from build123d import *

# Parameters (mm, degrees)
SKETCH1_W           = 40.9
SKETCH1_H           = 26.8
BOSS_EXTRUDE1_DEPTH = 10
SKETCH2_W           = 54
SKETCH2_H           = 20
BOSS_EXTRUDE2_DEPTH = 3
SKETCH3_R           = 1.5
CUT_EXTRUDE1_DEPTH  = 3
SKETCH4_W           = 40.9
SKETCH4_H           = 20
BOSS_EXTRUDE3_DEPTH = 3
BOSS_EXTRUDE4_DEPTH = 4.2
SKETCH6_R           = 2.5
BOSS_EXTRUDE5_DEPTH = 5


with BuildPart() as part:
    # Sketch1 → Boss-Extrude1 (new, symmetric)
    with BuildSketch(Plane.XY):
        Rectangle(SKETCH1_W, SKETCH1_H)
    extrude(amount=BOSS_EXTRUDE1_DEPTH, both=True)

    # Sketch2 → Boss-Extrude2 (add)
    with BuildSketch(Plane(origin=(0, 13.4, 0), x_dir=(1, 0, 0), z_dir=(0, 1, 0))):
        Rectangle(SKETCH2_W, SKETCH2_H)
    extrude(amount=BOSS_EXTRUDE2_DEPTH)

    # Sketch3 → Cut-Extrude1 (cut)
    with BuildSketch(Plane(origin=(0, 16.4, 0), x_dir=(1, 0, 0), z_dir=(0, 1, 0))):
        with Locations(Location((-24, 0, 0), (0, 0, 180))):
            Circle(SKETCH3_R)
        with Locations(Location((24, 0, 0), (0, 0, 180))):
            Circle(SKETCH3_R)
    extrude(amount=-CUT_EXTRUDE1_DEPTH, mode=Mode.SUBTRACT)

    # Sketch4 → Boss-Extrude3 (add)
    with BuildSketch(Plane(origin=(0, 16.4, 0), x_dir=(1, 0, 0), z_dir=(0, 1, 0))):
        Rectangle(SKETCH4_W, SKETCH4_H)
    extrude(amount=BOSS_EXTRUDE3_DEPTH)

    # Sketch5 → Boss-Extrude4 (add)
    with BuildSketch(Plane(origin=(0, 19.4, 0), x_dir=(1, 0, 0), z_dir=(0, 1, 0))):
        with BuildLine():
            ThreePointArc((0.870933014, -2.870797047), (20.45, 0), (0.870933014, 2.870797047))
            ThreePointArc((0.870933014, 2.870797047), (-3, 0), (0.870933014, -2.870797047))
        make_face()
    extrude(amount=BOSS_EXTRUDE4_DEPTH)

    # Sketch6 → Boss-Extrude5 (add)
    with BuildSketch(Plane(origin=(0, 23.6, 0), x_dir=(1, 0, 0), z_dir=(0, 1, 0))):
        with Locations(Location((10.45, 0, 0), (0, 0, 270))):
            Circle(SKETCH6_R)
    extrude(amount=BOSS_EXTRUDE5_DEPTH)


solid = part.part
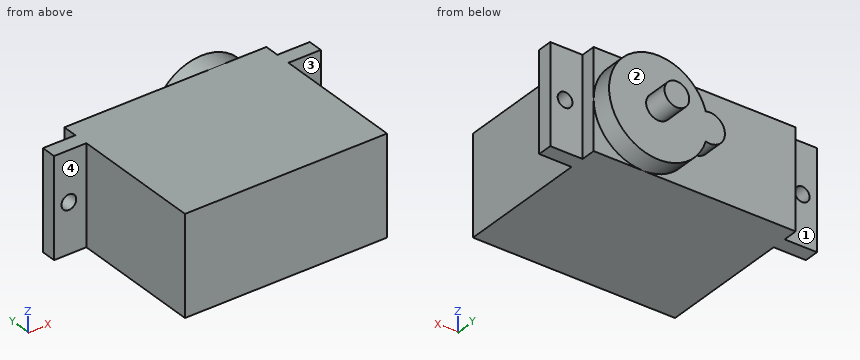
Can you work these out from the model? Positions are in its coordinate system, mm. Face numbers are marked on the shaded views. A direction names the side the tool comes from. Round coordinates to 2 decimals unless told otherwise and drop trailing zeros. Write each loop counter-clockwise with the first axis right and the second up, starting at its lowest first coordinate (ties: lowest second). Pieces come first, ordered by that corner, then holes. Notation, with made-up numbers: (-34, 84.5) -> (14, 84.5) arc R26 cw to (14, 99.5) -> close; hole circle Ø5 at (-23.75, -39.5). An arc over 180 degrees is marked (long way). One line per question, with ' | ' between items. Start each with the question number.
1) Suppose I cut it at D-D on y = 7. Write out the boundary of the cut face in (x, z), then the cut area to 3 significant figures.
2) I need wall thicknesses on line 1 (Z direction, x = 24, y = 14.95); line 2 (Y direction, x = 12, z = 4); line 3 (Y direction, x = 20, z = 9). Which ranges of each line are inside material? Lowest first, please. Write a range as [from, to].
3) I'm going to push flat-ended pins straight in: P1, Ø10, axis at y = 21, z = -1.5, coming from the +X side; P2, Ø7, axis at x = -25, z = -3.5, coming from the -Y side; P3, Ø5, axis at x = -22.5, z = 0, coming from the +Y side; P4, Ø0.9, axis at y = 17.5, z = 4.5, coming from the +X side. Where does each tip first touch, or does it pass through?
4) Suppose I cut it at A-A on x = 24. Write out the boundary of the cut face in (y, z), then the cut area to 3 significant figures.
5) Suppose I cut it at B-B on z = 4.75. Write out the boundary of the cut face in (x, y).
6) On a 3-axis mill with a long thin cutter (end or side, diameter ignored), from which of +Z, -Z, +X, -X, +Y, -Y can I reach the whole of each face in a straight line? I mean the marked faces 1, 2, 3 and 4. Say none if no direction works.
7) Suppose I cut it at C-C on x = 0. Write out the boundary of the cut face in (y, z), then the cut area to 3 significant figures.
Return value:
1) outline: (-20.45, -10) -> (20.45, -10) -> (20.45, 10) -> (-20.45, 10) -> close | area: 818 mm2
2) line 1: z = [-10, -1.5], [1.5, 10] | line 2: y = [-13.4, 23.6] | line 3: y = [-13.4, 19.4]
3) P1: stops at x = 27 | P2: stops at y = 13.4 | P3: stops at y = 19.4 | P4: stops at x = 20.45
4) outline: (13.4, -10) -> (16.4, -10) -> (16.4, -1.5) -> (13.4, -1.5) -> close; (13.4, 1.5) -> (16.4, 1.5) -> (16.4, 10) -> (13.4, 10) -> close | area: 51.0 mm2
5) outline: (-27, 13.4) -> (-20.45, 13.4) -> (-20.45, -13.4) -> (20.45, -13.4) -> (20.45, 13.4) -> (27, 13.4) -> (27, 16.4) -> (20.45, 16.4) -> (20.45, 19.4) -> (19.25, 19.4) -> (19.25, 23.6) -> (1.65, 23.6) -> (1.65, 19.4) -> (-20.45, 19.4) -> (-20.45, 16.4) -> (-27, 16.4) -> close
6) face 1: +Z, -Z, -X, +Y | face 2: +Y | face 3: +Z, -Z, +X, -Y | face 4: +Z, -Z, -X, -Y
7) outline: (-13.4, -10) -> (19.4, -10) -> (19.4, -3) -> (23.6, -3) -> (23.6, 3) -> (19.4, 3) -> (19.4, 10) -> (-13.4, 10) -> close | area: 681 mm2
